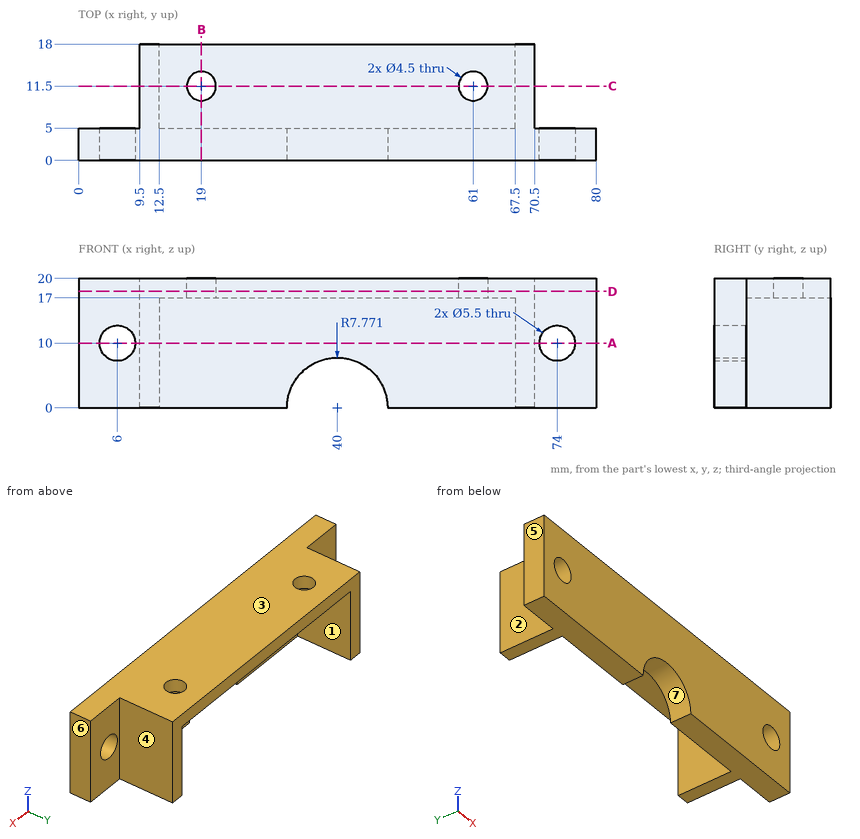
Study the drawing (mm; zero at the part's minimum x, y, z) and answer. A direction names the side the tool comes from. Give positions to 0.01 mm unless a question says otherwise; leave off trailing zeros. Loops run counter-clockwise (first coordinate to the right, second up) from the corner with the lowest first, then second, coordinate; pieces in that order, holes last. Notation, with made-up numbers: (-17, -32) - (11, -32) arc R20 cw to (11, -15) - close; hole circle Ø7 at (59, -27). An arc over 180 degrees is marked (long way). Use CSV: the item, a comma, the result in double quotes. Start each with the question number.
(1) Find section D-D, the plane z = 18. Determine the outline of the cut face in (x, y).
(2) Find section B-B, the plane x = 19. Determine the outline of the cut face in (y, z).
(3) Each of these flat-tipped pins is pushed along its axis until it touches: pin 1 (4 mm diameter, centred on x = 40, y = 14, fed in from -Z); pin 2 (7.5 mm diameter, centred on x = 4, z = 8.5, fed in from +Y); pin 3 (5 mm diameter, centred on x = 74, z = 10, fed in from -Y); pin 4 (4 mm diameter, centred on y = 9.5, z = 9.5, fed in from -X). Where does it stop, or does it pass through?
(4) Find section A-A, the plane z = 10. Determine the outline of the cut face in (x, y), plus the area to 3 significant figures.
(5) Find the intervals of material crossed by L1, parallel to Z at x = 6, y = 2.3; L2, parallel to Y at x = 61, z = 18.5; L3, parallel to X at y = 7.25, z = 3, in increasing order.
(6) A tool of negligible diameter and unlimited length cuts with its end or side. For the marked faces 1, 2, 3 and 4, from which of +Z, -Z, +X, -X, +Y, -Y can it reach the whole face along a straight path? Write none if from no direction.
(7) Find section C-C, the plane y = 11.5. Determine the outline of the cut face in (x, z), plus the area to 3 significant figures.
(8) Determine the mould class of the marked faces 5, 6 and 7 for opening direction X: released by +X, released by -X, zero draft, split by the parting line, or undercut.
Results found:
1,outline,"(0, 0) - (80, 0) - (80, 5) - (70.5, 5) - (70.5, 18) - (9.5, 18) - (9.5, 5) - (0, 5) - close; hole circle Ø4.5 at (19, 11.5); hole circle Ø4.5 at (61, 11.5)"
2,outline,"(0, 0) - (5, 0) - (5, 17) - (9.25, 17) - (9.25, 20) - (0, 20) - close; (13.75, 17) - (18, 17) - (18, 20) - (13.75, 20) - close"
3,pin 1,"z = 17"
3,pin 2,"y = 5"
3,pin 3,"through"
3,pin 4,"x = 9.5"
4,outline,"(0, 0) - (3.25, 0) - (3.25, 5) - (0, 5) - close; (8.75, 0) - (71.25, 0) - (71.25, 5) - (70.5, 5) - (70.5, 18) - (67.5, 18) - (67.5, 5) - (12.5, 5) - (12.5, 18) - (9.5, 18) - (9.5, 5) - (8.75, 5) - close; (76.75, 0) - (80, 0) - (80, 5) - (76.75, 5) - close"
4,area,"423 mm^2"
5,L1,"0 to 7.25, 12.75 to 20"
5,L2,"0 to 9.25, 13.75 to 18"
5,L3,"9.5 to 12.5, 67.5 to 70.5"
6,face 1,"-Z, +Y"
6,face 2,"+Z, -Z, -X, +Y"
6,face 3,"+Z, +X, -X, +Y, -Y"
6,face 4,"+Z, -Z, +X, +Y"
7,outline,"(9.5, 0) - (12.5, 0) - (12.5, 17) - (16.75, 17) - (16.75, 20) - (9.5, 20) - close; (21.25, 17) - (58.75, 17) - (58.75, 20) - (21.25, 20) - close; (63.25, 17) - (67.5, 17) - (67.5, 0) - (70.5, 0) - (70.5, 20) - (63.25, 20) - close"
7,area,"258 mm^2"
8,face 5,"released by -X"
8,face 6,"released by +X"
8,face 7,"undercut"
